The listing builds one solid part. Answer for the finished solid, in the listing's coordinates (mm). Face numbers are marked on the shaded views. A direction names the side the tool comes from. Coordinates: 2 decimals unless noted, no trailing zeros. Loops run counter-clockwise (first coordinate to the right, second up) from the corner with the lowest first, then second, coordinate; pieces in that order, holes last. Notation, with made-up numbers: M 74.25,-11 L 130.25,-11 A11 ccw 130.25,-1 Z; hole C 76,49.25 d3. An arc over 180 degrees is marked long. Answer as a JSON object with one key per item and string values. Group by question number.
1. A cutting plane is placed at B-B on x = -32.5. Give the vertices of the cut face in (y, z), and give its area (3 significant figures).
2. A cutting plane is placed at A-A on y = 14. Give the vertices of the cut face in (x, z).
3. Given pin 1 (1 mm diameter, centred on x = -45, y = 2.5, fed in from +Z); pin 2 (1.5 mm diameter, centred on x = -44, z = 0.5, fed in from +Y); pin 3 (1.5 mm diameter, centred on y = 22.5, z = 29.5, fed in from +X), each flat-ended and moving along its own axis, determine where each tip first touches the part or whether it passes through.
4. A cutting plane is placed at C-C on z = 39. Give the vertices of the cut face in (x, y), and give its area (3 significant figures).
5. Determine the mould class of the marked faces 1, 2 and 3 for opening direction X: released by +X, released by -X, zero draft, split by the parting line, or undercut.
6. Straight lines are drawn through the part: L1, parallel to X at y = 8.5, z = 54; L2, parallel to Y at x = -41.5, z = 8.5; L3, parallel to Y at x = -31, z = 17.5. For each, find the intervals that lie inside material, in ascending order.
7. For the marked faces 4, 5, 6 and 7, determine the directions among +Z, -Z, +X, -X, +Y, -Y from which every point of the face is accessible in a straight line to the end or side of a thin tool.
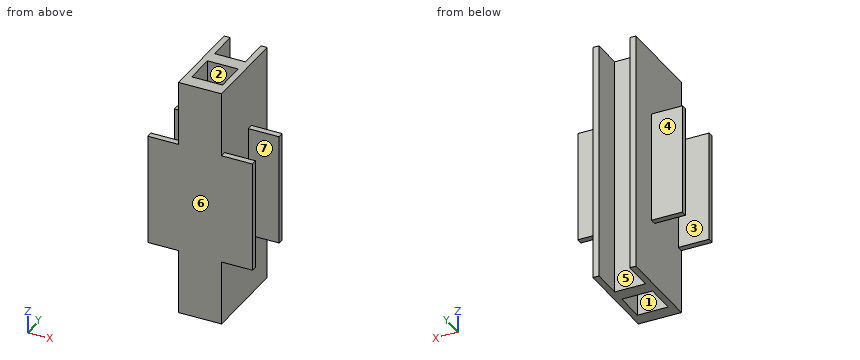
Autodesk Inventor part; units mm, degrees
ref_plane "YZ Plane" through (0, 0, 0) normal (1, 0, 0) x (0, 1, 0)
ref_plane "XZ Plane" through (0, 0, 0) normal (0, 1, 0) x (-1, 0, 0)
ref_plane "XY Plane" through (0, 0, 0) normal (0, 0, 1) x (1, 0, 0)
sketch "Sketch1" plane through (0, 0, 0) normal (0, 0, 1) x (1, 0, 0)
  line L0 (-36.8287, 15.6534) -> (-26.8287, 15.6534)
  line L1 (-26.8287, 15.6534) -> (-26.8287, 5.6534)
  line L2 (-26.8287, 5.6534) -> (-36.8287, 5.6534)
  line L3 (-36.8287, 5.6534) -> (-36.8287, 15.6534)
  line L4 (-31.8287, 15.6534) -> (-31.8287, 5.6534) construction
  line L5 (-31.8287, 20.1534) -> (-48.8287, 20.1534)
  line L6 (-48.8287, 20.1534) -> (-48.8287, 18.1534)
  line L7 (-48.8287, 18.1534) -> (-38.8287, 18.1534)
  line L8 (-38.8287, 18.1534) -> (-38.8287, 3.1534)
  line L9 (-38.8287, 3.1534) -> (-48.8287, 3.1534)
  line L10 (-48.8287, 3.1534) -> (-48.8287, 1.1534)
  line L11 (-48.8287, 1.1534) -> (-31.8287, 1.1534)
  line L12 (-36.8287, 10.6534) -> (-26.8287, 10.6534) construction
  line L13 (-31.8287, 20.1534) -> (-14.8287, 20.1534)
  line L14 (-14.8287, 20.1534) -> (-14.8287, 18.1534)
  line L15 (-14.8287, 18.1534) -> (-24.8287, 18.1534)
  line L16 (-24.8287, 18.1534) -> (-24.8287, 3.1534)
  line L17 (-24.8287, 3.1534) -> (-14.8287, 3.1534)
  line L18 (-14.8287, 3.1534) -> (-14.8287, 1.1534)
  line L19 (-14.8287, 1.1534) -> (-31.8287, 1.1534)
  dimension "d3" = 10
  dimension "d4" = 10
  dimension "d5" = 15
  dimension "d6" = 2
  dimension "d7" = 2
  dimension "d8" = 4.5
  dimension "d9" = 4.5
  dimension "d10" = 2
  dimension "d11" = 10
  dimension "d13" = 17
  dimension "d14" = 17
extrude "Extrusion1" add sketch "Sketch1" along normal blind 36
sketch "Sketch2" plane through (0, 0, 36) normal (0, 0, 1) x (1, 0, 0)
  line L0 (-36.8287, 5.6534) -> (-36.8287, 15.6534)
  line L1 (-26.8287, 5.6534) -> (-36.8287, 5.6534)
  line L2 (-36.8287, 15.6534) -> (-26.8287, 15.6534)
  line L3 (-26.8287, 15.6534) -> (-26.8287, 5.6534)
  line L4 (-26.8287, 5.6534) -> (-36.8287, 5.6534)
  line L5 (-36.8287, 5.6534) -> (-36.8287, 15.6534)
  line L6 (-38.8287, 20.1534) -> (-24.8287, 20.1534)
  line L7 (-24.8287, 20.1534) -> (-24.8287, 1.1534)
  line L8 (-24.8287, 1.1534) -> (-38.8287, 1.1534)
  line L9 (-38.8287, 1.1534) -> (-38.8287, 20.1534)
  line L10 (-14.8287, 20.1534) -> (-48.8287, 20.1534)
  point P0 (0, 0)
  dimension "d17" = 14
  dimension "d19" = 4.5
  dimension "d20" = 4.5
  dimension "d21" = 2
  dimension "d22" = 2
extrude "Extrusion2" add sketch "Sketch2" along normal blind 21
sketch "Sketch3" plane through (0, 0, 0) normal (0, 0, -1) x (-1, 0, 0)
  line L0 (26.8287, 5.6534) -> (26.8287, 15.6534)
  line L1 (36.8287, 5.6534) -> (26.8287, 5.6534)
  line L2 (26.8287, 15.6534) -> (36.8287, 15.6534)
  line L3 (36.8287, 15.6534) -> (36.8287, 5.6534)
  line L4 (36.8287, 5.6534) -> (26.8287, 5.6534)
  line L5 (26.8287, 5.6534) -> (26.8287, 15.6534)
  line L6 (24.8287, 20.1534) -> (38.8287, 20.1534)
  line L7 (38.8287, 20.1534) -> (38.8287, 1.1534)
  line L8 (38.8287, 1.1534) -> (24.8287, 1.1534)
  line L9 (24.8287, 1.1534) -> (24.8287, 20.1534)
  line L10 (49.3332, 20.1534) -> (15.3332, 20.1534)
  line L11 (36.8287, 15.6534) -> (26.8287, 15.6534)
  line L12 (26.8287, 5.6534) -> (36.8287, 5.6534)
  line L13 (36.8287, 5.6534) -> (36.8287, 15.6534)
  line L14 (26.8287, 15.6534) -> (26.8287, 5.6534)
  line L15 (14.8287, 20.1534) -> (48.8287, 20.1534)
  point P0 (0, 0)
  dimension "d25" = 14
  dimension "d26" = 4.5
  dimension "d27" = 4.5
  dimension "d28" = 2
  dimension "d29" = 2
extrude "Extrusion3" add sketch "Sketch3" along normal blind 21
sketch "Sketch4" plane through (0, 0, 57) normal (0, 0, 1) x (1, 0, 0)
  line L0 (-38.8287, 20.1534) -> (-48.8287, 20.1534)
  line L1 (-38.8287, 20.1534) -> (-38.8287, 30.1534)
  line L2 (-38.8287, 30.1534) -> (-36.8287, 30.1534)
  line L3 (-36.8287, 30.1534) -> (-36.8287, 20.1534)
  line L4 (-36.8287, 20.1534) -> (-26.8287, 20.1534)
  line L5 (-24.8287, 20.1534) -> (-38.8287, 20.1534)
  line L6 (-26.8287, 30.1534) -> (-24.8287, 30.1534)
  line L7 (-24.8287, 30.1534) -> (-24.8287, 20.1534)
  line L8 (-26.8287, 30.1534) -> (-26.8287, 20.1534)
  line L9 (-38.8287, 20.1534) -> (-38.8287, 1.1534)
  line L10 (-38.8287, 20.1534) -> (-36.8287, 20.1534)
  line L11 (-14.8287, 20.1534) -> (-24.8287, 20.1534)
  line L12 (-24.8287, 20.1534) -> (-26.8287, 20.1534)
  point P0 (0, 0)
  dimension "d32" = 2
  dimension "d33" = 2
  dimension "d34" = 10
extrude "Extrusion4" add sketch "Sketch4" against normal up to surface (78 mm away)
equation "\"d4\" = d3"
equation "\"d7\" = d6"
equation "\"d8\" = d9"
equation "\"d14\" = d13"
equation "\"d19\" = d20"
equation "\"d21\" = d22"
equation "\"d26\" = d27"
equation "\"d28\" = d29"
properties part number "fuselage_tail_interface_v2"
From the geometry:
{
 "1": {"outline": "M 1.15,-21 L 5.65,-21 L 5.65,57 L 1.15,57 Z; M 15.65,-21 L 20.15,-21 L 20.15,57 L 15.65,57 Z", "area": "702 mm²"},
 "2": {"outline": "M -38.83,-21 L -36.83,-21 L -36.83,57 L -38.83,57 Z; M -26.83,-21 L -24.83,-21 L -24.83,57 L -26.83,57 Z"},
 "3": {"pin 1": "stops at z = 36", "pin 2": "stops at y = 20.15", "pin 3": "stops at x = -24.83"},
 "4": {"outline": "M -38.83,1.15 L -24.83,1.15 L -24.83,30.15 L -26.83,30.15 L -26.83,20.15 L -36.83,20.15 L -36.83,30.15 L -38.83,30.15 Z; hole M -36.83,5.65 L -26.83,5.65 L -26.83,15.65 L -36.83,15.65 Z", "area": "206 mm²"},
 "5": {"face 1": "undercut", "face 2": "undercut", "face 3": "zero draft"},
 "6": {"L1": "x = -38.83 to -36.83, -26.83 to -24.83", "L2": "y = 1.15 to 3.15, 18.15 to 20.15", "L3": "y = 1.15 to 5.65, 15.65 to 20.15"},
 "7": {"face 4": "+Z, -Z, -X, +Y", "face 5": "+Z, -Z, +Y", "face 6": "+Z, -Z, +X, -X, -Y", "face 7": "+Z, -Z, +X"}
}
